Check sheet for the drawn part. Datum: minimum x, y, z corner. Units: mm. A direction names the side the tool comes from. Coordinates: 2 decimals unless noted, no trailing zeros. Write each loop counter-clockwise with the first axis right and the second up, starting at its lowest first coordinate (ties: lowest second). Pieces come first, ordered by that corner, then holes. Notation, with made-up numbers: M 1.25,16.5 L 23.25,16.5 A23 cw 23.25,26.5 Z; hole C -39.5,74.25 d5. An arc over 180 degrees is marked long. Answer as CSV lines item,"result". Start each with the question number.
Q1. Thickness scan on line 1 along Y through (x, z) = (30, 78.25); line 2 along Z through (x, y) = (44, 29); line 3 along Z through (x, y) = (42.5, 52.5). Record the ranges inside material, lowest first. Write a range as from..to.
Q2. Sectioned sample at D-D, the plane z = 71. Record the cut outline in (x, y).
Q3. Sectioned sample at A-A, the plane z = 81. Record the cut outline in (x, y) (1 decimal).
Q4. Sectioned sample at B-B, the plane x = 30. Record the cut outline in (y, z), then the cut area to 3 significant figures.
Q5. Access from +Z, -Z, +X, -X, +Y, -Y to the whole of each face (thin tool, end or side, straight path). Record for the marked faces 1, 2 and 3.
Q6. Sectioned sample at C-C, the plane y = 30. Record the cut outline in (x, z).
Q7. Depth check by flat-ended pin: pin 1 Ø10 at (y, z) = (41.5, 24) entering from +X; pin 2 Ø10 at (x, y) = (22.5, 41) entering from +Z; pin 3 Ø7 at (x, y) = (41.5, 52.5) entering from +Z; pin 4 Ø12 at (x, y) = (20.5, 49) entering from +Z. Enter the tip coordinate at first touch or a pass-through.
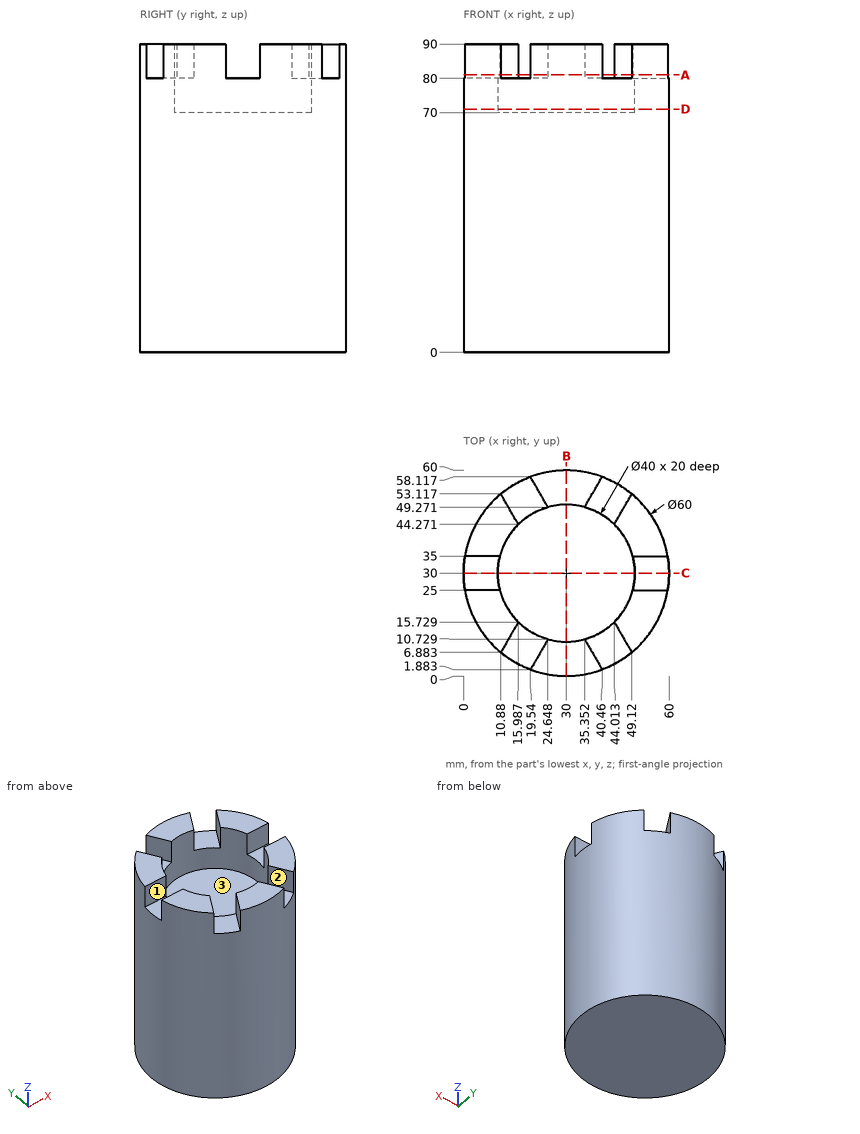
Output:
1,line 1,"y = 0..10, 50..60"
1,line 2,"z = 0..70"
1,line 3,"z = 0..80"
2,outline,"C 30,30 d60; hole C 30,30 d40"
3,outline,"M 0.4,25 A30 ccw 10.9,6.9 L 16,15.7 A20 cw 10.6,25 Z; M 0.4,35 L 10.6,35 A20 cw 16,44.3 L 10.9,53.1 A30 ccw Z; M 19.5,1.9 A30 ccw 40.5,1.9 L 35.4,10.7 A20 cw 24.6,10.7 Z; M 19.5,58.1 L 24.6,49.3 A20 cw 35.4,49.3 L 40.5,58.1 A30 ccw Z; M 44,15.7 L 49.1,6.9 A30 ccw 59.6,25 L 49.4,25 A20 cw Z; M 44,44.3 A20 cw 49.4,35 L 59.6,35 A30 ccw 49.1,53.1 Z"
4,outline,"M 0,0 L 60,0 L 60,90 L 50,90 L 50,70 L 10,70 L 10,90 L 0,90 Z"
4,area,"4,600 mm^2"
5,face 1,"+Z, +X, -X"
5,face 2,"+Z, -Y"
5,face 3,"+Z"
6,outline,"M 0,0 L 60,0 L 60,80 L 50,80 L 50,70 L 10,70 L 10,80 L 0,80 Z"
7,pin 1,"stops at x = 59.29"
7,pin 2,"stops at z = 70"
7,pin 3,"stops at z = 80"
7,pin 4,"stops at z = 90"
